For this review, take the finished solid that the model builds, in its own axes (mm). Coordinates: 2 decimals unless noted, no trailing zeros. Loops run counter-clockwise (first coordinate to the right, second up) from the corner with the lowest first, then second, coordinate; pieces in that order, holes last. Notation, with made-up numbers: M 80.25,88.5 L 120.25,88.5 A14 cw 120.25,104.5 Z; hole C 38.25,-5.75 d11. An arc over 180 degrees is marked long. Write item = value, one per line.
from build123d import *

# Parameters (mm, degrees)
RESSALTO_EXTRUS_O1_DEPTH = 5
CORTE_EXTRUS_O1_DEPTH    = 5
ESBO_O3_W                = 5
ESBO_O3_H                = 17
CORTE_EXTRUS_O3_DEPTH    = 5
CORTE_EXTRUS_O4_DEPTH    = 10
CORTE_EXTRUS_O5_DEPTH    = 5
ESBO_O6_R                = 1.5
CORTE_EXTRUS_O6_DEPTH    = 20
CORTE_EXTRUS_O7_DEPTH    = 10


with BuildPart() as part:
    # Esboço1 → Ressalto-extrusão1 (new body)
    with BuildSketch(Plane(origin=(0, 0, 0), x_dir=(1, 0, 0), z_dir=(0, 1, 0))):
        with BuildLine():
            Line((-56.5, -61.5), (56.5, -61.5))
            ThreePointArc((56.5, -61.5), (60.035533906, -60.035533906), (61.5, -56.5))
            Line((61.5, -56.5), (61.5, 56.5))
            ThreePointArc((61.5, 56.5), (60.035533906, 60.035533906), (56.5, 61.5))
            Line((56.5, 61.5), (-56.5, 61.5))
            ThreePointArc((-56.5, 61.5), (-60.035533906, 60.035533906), (-61.5, 56.5))
            Line((-61.5, 56.5), (-61.5, -56.5))
            ThreePointArc((-61.5, -56.5), (-60.035533906, -60.035533906), (-56.5, -61.5))
        make_face()
    extrude(amount=RESSALTO_EXTRUS_O1_DEPTH)

    # Esboço2 → Corte-extrusão1 (cut)
    with BuildSketch(Plane(origin=(0, 5, 0), x_dir=(1, 0, 0), z_dir=(0, 1, 0))):
        with BuildLine():
            Line((1.233117681, 54.5), (-1.233117681, 54.5))
            ThreePointArc((-1.233117681, 54.5), (-2.48249215, 53.98249215), (-3, 52.733117681))
            Line((-3, 52.733117681), (-3, 40.733117681))
            ThreePointArc((-3, 40.733117681), (-2.48249215, 39.483743212), (-1.233117681, 38.966235362))
            Line((-1.233117681, 38.966235362), (1.233117681, 38.966235362))
            ThreePointArc((1.233117681, 38.966235362), (2.48249215, 39.483743212), (3, 40.733117681))
            Line((3, 40.733117681), (3, 52.733117681))
            ThreePointArc((3, 52.733117681), (2.48249215, 53.98249215), (1.233117681, 54.5))
        make_face()
        with BuildLine():
            Line((-7.266882319, 54.5), (-9.733117681, 54.5))
            ThreePointArc((-9.733117681, 54.5), (-10.98249215, 53.98249215), (-11.5, 52.733117681))
            Line((-11.5, 52.733117681), (-11.5, 40.733117681))
            ThreePointArc((-11.5, 40.733117681), (-10.98249215, 39.483743212), (-9.733117681, 38.966235362))
            Line((-9.733117681, 38.966235362), (-7.266882319, 38.966235362))
            ThreePointArc((-7.266882319, 38.966235362), (-6.01750785, 39.483743212), (-5.5, 40.733117681))
            Line((-5.5, 40.733117681), (-5.5, 52.733117681))
            ThreePointArc((-5.5, 52.733117681), (-6.01750785, 53.98249215), (-7.266882319, 54.5))
        make_face()
        with BuildLine():
            Line((7.266882319, 38.966235362), (9.733117681, 38.966235362))
            ThreePointArc((9.733117681, 38.966235362), (10.98249215, 39.483743212), (11.5, 40.733117681))
            Line((11.5, 40.733117681), (11.5, 52.733117681))
            ThreePointArc((11.5, 52.733117681), (10.98249215, 53.98249215), (9.733117681, 54.5))
            Line((9.733117681, 54.5), (7.266882319, 54.5))
            ThreePointArc((7.266882319, 54.5), (6.01750785, 53.98249215), (5.5, 52.733117681))
            Line((5.5, 52.733117681), (5.5, 40.733117681))
            ThreePointArc((5.5, 40.733117681), (6.01750785, 39.483743212), (7.266882319, 38.966235362))
        make_face()
    extrude(amount=-CORTE_EXTRUS_O1_DEPTH, mode=Mode.SUBTRACT)

    # Esboço3 → Corte-extrusão3 (cut)
    with BuildSketch(Plane(origin=(0, 5, 0), x_dir=(1, 0, 0), z_dir=(0, 1, 0))):
        with Locations((-59, -34)):
            Rectangle(ESBO_O3_W, ESBO_O3_H)
        with Locations((59, -34)):
            Rectangle(ESBO_O3_W, ESBO_O3_H)
    extrude(amount=-CORTE_EXTRUS_O3_DEPTH, mode=Mode.SUBTRACT)

    # Esboço4 → Corte-extrusão4 (cut)
    with BuildSketch(Plane(origin=(0, 5, 0), x_dir=(1, 0, 0), z_dir=(0, 1, 0))):
        Polygon((56.5, -41.5), (53, -41.5), (53, -43.3), (51.5, -43.3), (51.5, -41.5), (49.5, -41.5), (49.5, -39.5), (51.5, -39.5), (51.5, -37.7), (53, -37.7), (53, -39.5), (56.5, -39.5), align=None)
        Polygon((56.5, -26.5), (53, -26.5), (53, -24.7), (51.5, -24.7), (51.5, -26.5), (49.5, -26.5), (49.5, -28.5), (51.5, -28.5), (51.5, -30.3), (53, -30.3), (53, -28.5), (56.5, -28.5), align=None)
    corte_extrus_o4 = extrude(amount=-CORTE_EXTRUS_O4_DEPTH, mode=Mode.SUBTRACT)

    # Espelhar1: Corte-extrusão4 across plane
    add(corte_extrus_o4.mirror(Plane(origin=(0, 0, 0), x_dir=(0, 0, 1), z_dir=(1, 0, 0))), mode=Mode.SUBTRACT)

    # Esboço5 → Corte-extrusão5 (cut)
    with BuildSketch(Plane(origin=(0, 5, 0), x_dir=(1, 0, 0), z_dir=(0, 1, 0))):
        with BuildLine():
            Line((43, -42.5), (-43, -42.5))
            ThreePointArc((-43, -42.5), (-44.414213562, -41.914213562), (-45, -40.5))
            Line((-45, -40.5), (-45, -28.5))
            ThreePointArc((-45, -28.5), (-44.414213562, -27.085786438), (-43, -26.5))
            Line((-43, -26.5), (43, -26.5))
            ThreePointArc((43, -26.5), (44.414213562, -27.085786438), (45, -28.5))
            Line((45, -28.5), (45, -40.5))
            ThreePointArc((45, -40.5), (44.414213562, -41.914213562), (43, -42.5))
        make_face()
    extrude(amount=-CORTE_EXTRUS_O5_DEPTH, mode=Mode.SUBTRACT)

    # Esboço6 → Corte-extrusão6 (cut)
    with BuildSketch(Plane(origin=(0, 5, 0), x_dir=(1, 0, 0), z_dir=(0, 1, 0))):
        with Locations(Location((-51.5, 46.5, 0), (0, 0, 270))):
            Circle(ESBO_O6_R)
        with Locations(Location((51.5, 46.5, 0), (0, 0, 270))):
            Circle(ESBO_O6_R)
        with Locations(Location((31.75, -47.5, 0), (0, 0, 270))):
            Circle(ESBO_O6_R)
        with Locations(Location((-31.75, -47.5, 0), (0, 0, 270))):
            Circle(ESBO_O6_R)
    extrude(amount=-CORTE_EXTRUS_O6_DEPTH, mode=Mode.SUBTRACT)

    # Esboço7 → Corte-extrusão7 (cut)
    with BuildSketch(Plane.XZ):
        with BuildLine():
            Line((7.5, 61.5), (-7.5, 61.5))
            Line((-7.5, 61.5), (-7.5, 56.5))
            ThreePointArc((-7.5, 56.5), (-6.621320344, 54.378679656), (-4.5, 53.5))
            Line((-4.5, 53.5), (4.5, 53.5))
            ThreePointArc((4.5, 53.5), (6.621320344, 54.378679656), (7.5, 56.5))
            Line((7.5, 56.5), (7.5, 61.5))
        make_face()
    extrude(amount=-CORTE_EXTRUS_O7_DEPTH, mode=Mode.SUBTRACT)


solid = part.part
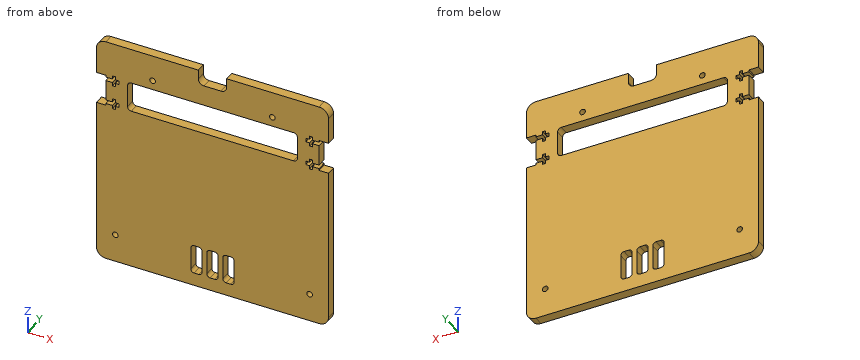
Q1. For line 1 along Z through (x, y) = (56, 4.7); line 2 along X through (y, z) = (3.8, 47.5); line 3 along X through (y, z) = (1.3, -43), list the stretches that pass through material, from the lowest coordinate up.
Solved:
line_1 = -61.5 to 26.5, 28.5 to 39.5, 41.5 to 61.5
line_2 = -61.5 to -33.25, -30.25 to 30.25, 33.25 to 61.5
line_3 = -61.5 to -11.5, -5.5 to -3, 3 to 5.5, 11.5 to 61.5
Q2. Add section A-A (x = -13). Write out the cut boundary in (y, z).
Solved:
outline = M 0,-61.5 L 5,-61.5 L 5,26.5 L 0,26.5 Z; M 0,42.5 L 5,42.5 L 5,61.5 L 0,61.5 Z
Q3. For pin 1 Ø1.4 at (y, z) = (1.5, 38.5) entering from +X; pin 2 Ø2.5 at (y, z) = (2, 59) entering from -X; pin 3 Ø2.5 at (x, y) = (-58, 1.5) entering from -Z; pin 4 Ø2 at (x, z) = (35, 22.5) entering from -Y, all flat-tipped, find the tip position at first contact; note any pin that passes through.
Solved:
pin_1 = 56.5
pin_2 = -61.34
pin_3 = -61.49
pin_4 = 0
Q4. Add section B-B (x = 31.75). Write out the cut boundary in (y, z), and give its area (3 significant figures).
Solved:
outline = M 0,-61.5 L 5,-61.5 L 5,26.5 L 0,26.5 Z; M 0,42.5 L 5,42.5 L 5,46 L 0,46 Z; M 0,49 L 5,49 L 5,61.5 L 0,61.5 Z
area = 520 mm²
Q5. Add section C-C (y = 1.75). State how many separate pieces and enclosed holes the cut face has, and give its area (3 significant figures).
Solved:
separate_pieces = 1
enclosed_holes = 8
area = 13,000 mm²
